CAD build for the part. Positions are in the model's coordinates, mm. A direction names the side the tool comes from. Round coordinates to 2 decimals unless told otherwise and drop trailing zeros. Order: outer loops, then holes, each group sorted by start corner. A loop starts at its lowest first (then second) coordinate and runs counter-clockwise, first axis right, second up. Notation, with made-up numbers: (65, 73.25) -> (97, 73.25) arc R11 ccw to (97, 93.25) -> close; hole circle Ø4 at (-33.75, 41). An arc over 180 degrees is marked (long way). Return JSON: item names as keys, results as strings. Group by question number.
Q1. Which spindle directions (+Z, -Z, +X, -X, +Y, -Y) get a long thin tool onto all of the face, cutting with end or side? Do faces 1 (the cylindrical face through (17.282, -8.334, 31.876)), 2 (the cylindrical face through (-0.776, -3.495, 7.331)). Say none if no direction does.
Q2. Probe line 1 along Y through (x, z) = (0, 7) (3 decimals); line 2 along X through (y, z) = (1.25, 19); line 3 along Y through (x, z) = (31, 29.5). List the from-to ranges inside material, lowest first.
Q3. Flat gauge pins, fed straight in: pin 1 (10 mm diameter, centred on y = 2.5, z = 25.5, fed in from -X); pin 2 (8 mm diameter, centred on y = -4, z = 13.5, fed in from +X); pin 3 (6 mm diameter, centred on x = 18, y = -10, fed in from -Z); pin 4 (4 mm diameter, centred on y = 1.5, z = 13.5, fed in from -X) (3 decimals). Where does each tip first touch, or does it go through?
Q4. Mould opens along X. For faces 3 (the flat face through (1, 4, 0)), 4 (the cylindrical face through (49.21, -12.09, 26.07)) say: +X half, -X half, draft (parallel to the pull), parting line (faces both ways), or undercut.
Q5. Cut at B-B (z = 10). Write the cut outline in (x, y) (3 decimals).
Q6. Cut at A-A (z = 16). Count the separate pieces of the cut face and the enclosed holes in it, then the cut area to 3 significant figures.
from build123d import *

# Parameters (mm, degrees)
SKETCH_1_R   = 4.765
SKETCH_1_R_2 = 3.58


with BuildPart() as part:
    # По траектории1: sweep along a curve in space
    with BuildLine() as sweep_1_path:
        Line((0, 0, 0), (0, 0, 14.460504946))
        ThreePointArc((17.378248064, -5.734487139, 34.388118956), (5.003679185, -1.651117755, 27.988232477), (0, 0, 14.460504946))
        Line((18.324445146, -6.046713952, 34.473121895), (17.378248064, -5.734487139, 34.388118956))
        ThreePointArc((29.914415781, -8, 32.362570038), (24.180183472, -7.500284638, 34.192857359), (18.324445146, -6.046713952, 34.473121895))
        Line((29.914415781, -8, 32.362570038), (65.938376067, -8, 15.576419335))
    # Эскиз1 → По траектории1 (sweep)
    with BuildSketch(Plane.XY):
        Circle(SKETCH_1_R)
        Circle(SKETCH_1_R_2, mode=Mode.SUBTRACT)
    sweep(path=sweep_1_path.line)


solid = part.part
Solution:
{
 "1": {"face 1": "none", "face 2": "-Z"},
 "2": {"line 1": "y = -4.765 to -3.58, 3.58 to 4.765", "line 2": "x = -4.16 to -2.88, 3.85 to 5.16", "line 3": "y = -12.26 to -10.87, -5.13 to -3.74"},
 "3": {"pin 1": "stops at x = -3.89", "pin 2": "stops at x = 66.83", "pin 3": "stops at z = 29.8", "pin 4": "stops at x = -4.765"},
 "4": {"face 3": "draft", "face 4": "undercut"},
 "5": {"outline": "circle Ø9.53 at (0, 0); hole circle Ø7.16 at (0, 0)"},
 "6": {"separate pieces": "2", "enclosed holes": "1", "area": "70.6 mm²"}
}
